The model under review builds one solid part; all positions refer to its coordinate system, in mm. Round coordinates to 2 decimals unless told otherwise and drop trailing zeros. Write each question's results on one line, items separated by ' | '. Start each with the question number.
Item 1: For L1, parallel to Y at x = 0, z = 259; L2, parallel to X at y = -1.75, z = 143.5; L3, parallel to X at y = 9, z = 249, list the stretches that pass through material, from the lowest coordinate up. Write a range as from..to.
Item 2: Clearance check with flat-ended pins moving along their axes: pin 1 Ø2 at (x, z) = (25.5, 328) entering from -Y; pin 2 Ø3 at (y, z) = (0, 280) entering from +X; pin 3 Ø1 at (x, y) = (3, -9) entering from +Z; pin 4 Ø0.7 at (y, z) = (-11.5, 204) entering from -X. State where each tip first meets the part, or that it passes through.
Item 3: We need section A-A (z = 344). Give the number of separate pieces and of enclosed holes in the cut face, and give its area (3 significant figures).
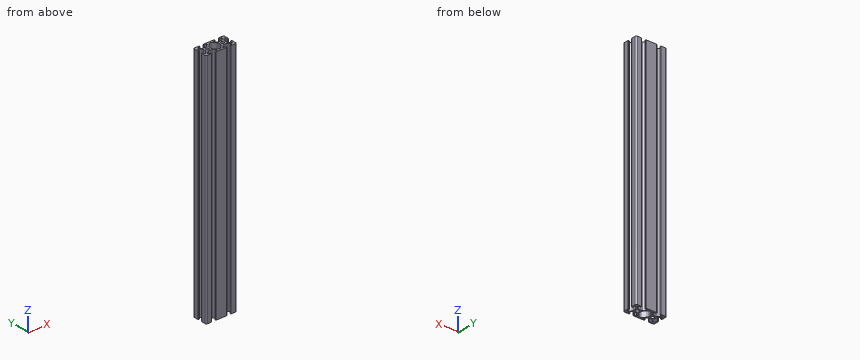
from build123d import *

# Parameters (mm, degrees)
SKETCH1_R           = 2.5527
BOSS_EXTRUDE1_DEPTH = 394.716


with BuildPart() as part:
    # Sketch1 → Boss-Extrude1 (new body)
    with BuildSketch(Plane.XY):
        with BuildLine():
            Line((-7.499820068, 9.062384633), (-4.117171405, 5.67973597))
            ThreePointArc((-4.117171405, 5.67973597), (-3.087127272, 4.991482484), (-1.872107374, 4.7498))
            Line((-1.872107374, 4.7498), (1.872107374, 4.7498))
            ThreePointArc((1.872107374, 4.7498), (3.087127272, 4.991482484), (4.117171405, 5.67973597))
            Line((4.117171405, 5.67973597), (7.499820068, 9.062384633))
            ThreePointArc((7.499820068, 9.062384633), (7.665000904, 9.892804775), (6.9610047, 10.3632))
            Line((6.9610047, 10.3632), (4.064, 10.3632))
            ThreePointArc((4.064, 10.3632), (3.525184633, 10.586384633), (3.302, 11.1252))
            Line((3.302, 11.1252), (3.302, 11.938))
            ThreePointArc((3.302, 11.938), (3.525184633, 12.476815367), (4.064, 12.7))
            Line((4.064, 12.7), (10.668, 12.7))
            Line((10.668, 12.7), (14.732, 12.7))
            Line((14.732, 12.7), (21.336, 12.7))
            ThreePointArc((21.336, 12.7), (21.874815367, 12.476815367), (22.098, 11.938))
            Line((22.098, 11.938), (22.098, 11.1252))
            ThreePointArc((22.098, 11.1252), (21.874815367, 10.586384633), (21.336, 10.3632))
            Line((21.336, 10.3632), (18.4389953, 10.3632))
            ThreePointArc((18.4389953, 10.3632), (17.734999096, 9.892804775), (17.900179932, 9.062384633))
            Line((17.900179932, 9.062384633), (21.282828595, 5.67973597))
            ThreePointArc((21.282828595, 5.67973597), (22.312872728, 4.991482484), (23.527892626, 4.7498))
            Line((23.527892626, 4.7498), (27.272107374, 4.7498))
            ThreePointArc((27.272107374, 4.7498), (28.487127272, 4.991482484), (29.517171405, 5.67973597))
            Line((29.517171405, 5.67973597), (32.899820068, 9.062384633))
            ThreePointArc((32.899820068, 9.062384633), (33.065000904, 9.892804775), (32.3610047, 10.3632))
            Line((32.3610047, 10.3632), (29.464, 10.3632))
            ThreePointArc((29.464, 10.3632), (28.925184633, 10.586384633), (28.702, 11.1252))
            Line((28.702, 11.1252), (28.702, 11.938))
            ThreePointArc((28.702, 11.938), (28.925184633, 12.476815367), (29.464, 12.7))
            Line((29.464, 12.7), (36.068, 12.7))
            ThreePointArc((36.068, 12.7), (37.504840979, 12.104840979), (38.1, 10.668))
            Line((38.1, 10.668), (38.1, 4.064))
            ThreePointArc((38.1, 4.064), (37.876815367, 3.525184633), (37.338, 3.302))
            Line((37.338, 3.302), (36.5252, 3.302))
            ThreePointArc((36.5252, 3.302), (35.986384633, 3.525184633), (35.7632, 4.064))
            Line((35.7632, 4.064), (35.7632, 6.9610047))
            ThreePointArc((35.7632, 6.9610047), (35.292804775, 7.665000904), (34.462384633, 7.499820068))
            Line((34.462384633, 7.499820068), (31.07973597, 4.117171405))
            ThreePointArc((31.07973597, 4.117171405), (30.391482484, 3.087127272), (30.1498, 1.872107374))
            Line((30.1498, 1.872107374), (30.1498, -1.872107374))
            ThreePointArc((30.1498, -1.872107374), (30.391482484, -3.087127272), (31.07973597, -4.117171405))
            Line((31.07973597, -4.117171405), (34.462384633, -7.499820068))
            ThreePointArc((34.462384633, -7.499820068), (35.292804775, -7.665000904), (35.7632, -6.9610047))
            Line((35.7632, -6.9610047), (35.7632, -4.064))
            ThreePointArc((35.7632, -4.064), (35.986384633, -3.525184633), (36.5252, -3.302))
            Line((36.5252, -3.302), (37.338, -3.302))
            ThreePointArc((37.338, -3.302), (37.876815367, -3.525184633), (38.1, -4.064))
            Line((38.1, -4.064), (38.1, -10.668))
            ThreePointArc((38.1, -10.668), (37.504840979, -12.104840979), (36.068, -12.7))
            Line((36.068, -12.7), (29.464, -12.7))
            ThreePointArc((29.464, -12.7), (28.925184633, -12.476815367), (28.702, -11.938))
            Line((28.702, -11.938), (28.702, -11.1252))
            ThreePointArc((28.702, -11.1252), (28.925184633, -10.586384633), (29.464, -10.3632))
            Line((29.464, -10.3632), (32.3610047, -10.3632))
            ThreePointArc((32.3610047, -10.3632), (33.065000904, -9.892804775), (32.899820068, -9.062384633))
            Line((32.899820068, -9.062384633), (29.517171405, -5.67973597))
            ThreePointArc((29.517171405, -5.67973597), (28.487127272, -4.991482484), (27.272107374, -4.7498))
            Line((27.272107374, -4.7498), (23.527892626, -4.7498))
            ThreePointArc((23.527892626, -4.7498), (22.312872728, -4.991482484), (21.282828595, -5.67973597))
            Line((21.282828595, -5.67973597), (17.900179932, -9.062384633))
            ThreePointArc((17.900179932, -9.062384633), (17.734999096, -9.892804775), (18.4389953, -10.3632))
            Line((18.4389953, -10.3632), (21.336, -10.3632))
            ThreePointArc((21.336, -10.3632), (21.874815367, -10.586384633), (22.098, -11.1252))
            Line((22.098, -11.1252), (22.098, -11.938))
            ThreePointArc((22.098, -11.938), (21.874815367, -12.476815367), (21.336, -12.7))
            Line((21.336, -12.7), (14.732, -12.7))
            Line((14.732, -12.7), (10.668, -12.7))
            Line((10.668, -12.7), (4.064, -12.7))
            ThreePointArc((4.064, -12.7), (3.525184633, -12.476815367), (3.302, -11.938))
            Line((3.302, -11.938), (3.302, -11.1252))
            ThreePointArc((3.302, -11.1252), (3.525184633, -10.586384633), (4.064, -10.3632))
            Line((4.064, -10.3632), (6.9610047, -10.3632))
            ThreePointArc((6.9610047, -10.3632), (7.665000904, -9.892804775), (7.499820068, -9.062384633))
            Line((7.499820068, -9.062384633), (4.117171405, -5.67973597))
            ThreePointArc((4.117171405, -5.67973597), (3.087127272, -4.991482484), (1.872107374, -4.7498))
            Line((1.872107374, -4.7498), (-1.872107374, -4.7498))
            ThreePointArc((-1.872107374, -4.7498), (-3.087127272, -4.991482484), (-4.117171405, -5.67973597))
            Line((-4.117171405, -5.67973597), (-7.499820068, -9.062384633))
            ThreePointArc((-7.499820068, -9.062384633), (-7.665000904, -9.892804775), (-6.9610047, -10.3632))
            Line((-6.9610047, -10.3632), (-4.064, -10.3632))
            ThreePointArc((-4.064, -10.3632), (-3.525184633, -10.586384633), (-3.302, -11.1252))
            Line((-3.302, -11.1252), (-3.302, -11.938))
            ThreePointArc((-3.302, -11.938), (-3.525184633, -12.476815367), (-4.064, -12.7))
            Line((-4.064, -12.7), (-10.668, -12.7))
            ThreePointArc((-10.668, -12.7), (-12.104840979, -12.104840979), (-12.7, -10.668))
            Line((-12.7, -10.668), (-12.7, -4.064))
            ThreePointArc((-12.7, -4.064), (-12.476815367, -3.525184633), (-11.938, -3.302))
            Line((-11.938, -3.302), (-11.1252, -3.302))
            ThreePointArc((-11.1252, -3.302), (-10.586384633, -3.525184633), (-10.3632, -4.064))
            Line((-10.3632, -4.064), (-10.3632, -6.9610047))
            ThreePointArc((-10.3632, -6.9610047), (-9.892804775, -7.665000904), (-9.062384633, -7.499820068))
            Line((-9.062384633, -7.499820068), (-5.67973597, -4.117171405))
            ThreePointArc((-5.67973597, -4.117171405), (-4.991482484, -3.087127272), (-4.7498, -1.872107374))
            Line((-4.7498, -1.872107374), (-4.7498, 1.872107374))
            ThreePointArc((-4.7498, 1.872107374), (-4.991482484, 3.087127272), (-5.67973597, 4.117171405))
            Line((-5.67973597, 4.117171405), (-9.062384633, 7.499820068))
            ThreePointArc((-9.062384633, 7.499820068), (-9.892804775, 7.665000904), (-10.3632, 6.9610047))
            Line((-10.3632, 6.9610047), (-10.3632, 4.064))
            ThreePointArc((-10.3632, 4.064), (-10.586384633, 3.525184633), (-11.1252, 3.302))
            Line((-11.1252, 3.302), (-11.938, 3.302))
            ThreePointArc((-11.938, 3.302), (-12.476815367, 3.525184633), (-12.7, 4.064))
            Line((-12.7, 4.064), (-12.7, 10.668))
            ThreePointArc((-12.7, 10.668), (-12.104840979, 12.104840979), (-10.668, 12.7))
            Line((-10.668, 12.7), (-4.064, 12.7))
            ThreePointArc((-4.064, 12.7), (-3.525184633, 12.476815367), (-3.302, 11.938))
            Line((-3.302, 11.938), (-3.302, 11.1252))
            ThreePointArc((-3.302, 11.1252), (-3.525184633, 10.586384633), (-4.064, 10.3632))
            Line((-4.064, 10.3632), (-6.9610047, 10.3632))
            ThreePointArc((-6.9610047, 10.3632), (-7.665000904, 9.892804775), (-7.499820068, 9.062384633))
        make_face()
        with Locations(Location((0, 0, 0), (0, 0, 180))):
            Circle(SKETCH1_R, mode=Mode.SUBTRACT)
        with Locations(Location((25.4, 0, 0), (0, 0, 180))):
            Circle(SKETCH1_R, mode=Mode.SUBTRACT)
        with BuildLine():
            Line((4.7498, -1.872107374), (4.7498, 1.872107374))
            ThreePointArc((4.7498, 1.872107374), (4.991482484, 3.087127272), (5.67973597, 4.117171405))
            Line((5.67973597, 4.117171405), (11.263159021, 9.700594456))
            ThreePointArc((11.263159021, 9.700594456), (12.7, 10.295753476), (14.136840979, 9.700594456))
            Line((14.136840979, 9.700594456), (19.72026403, 4.117171405))
            ThreePointArc((19.72026403, 4.117171405), (20.408517516, 3.087127272), (20.6502, 1.872107374))
            Line((20.6502, 1.872107374), (20.6502, -1.872107374))
            ThreePointArc((20.6502, -1.872107374), (20.408517516, -3.087127272), (19.72026403, -4.117171405))
            Line((19.72026403, -4.117171405), (14.136840979, -9.700594456))
            ThreePointArc((14.136840979, -9.700594456), (12.7, -10.295753476), (11.263159021, -9.700594456))
            Line((11.263159021, -9.700594456), (5.67973597, -4.117171405))
            ThreePointArc((5.67973597, -4.117171405), (4.991482484, -3.087127272), (4.7498, -1.872107374))
        make_face(mode=Mode.SUBTRACT)
    extrude(amount=BOSS_EXTRUDE1_DEPTH)


solid = part.part
Here are the results:
1) L1: y = -4.75..-2.55, 2.55..4.75 | L2: x = -4.75..-1.86, 1.86..4.75, 20.65..23.54, 27.26..30.15 | L3: x = -12.7..-7.44, 7.44..10.56, 14.84..17.96, 32.84..38.1
2) pin 1: stops at y = -4.75 | pin 2: stops at x = 30.15 | pin 3: passes through | pin 4: stops at x = -12.64
3) separate pieces: 1 | enclosed holes: 3 | area: 533 mm2
